```python
from build123d import *

# Parameters (mm, degrees)
SKETCH1_W           = 90
SKETCH1_H           = 45
BOSS_EXTRUDE1_DEPTH = 50
SKETCH2_R           = 4.15
CUT_EXTRUDE1_DEPTH  = 28.296664924
SKETCH3_R           = 4.15
CUT_EXTRUDE2_DEPTH  = 106.386194542


with BuildPart() as part:
    # Sketch1 → Boss-Extrude1 (new body)
    with BuildSketch(Plane(origin=(0, 0, 0), x_dir=(1, 0, 0), z_dir=(0, 1, 0))):
        Rectangle(SKETCH1_W, SKETCH1_H)
    extrude(amount=BOSS_EXTRUDE1_DEPTH)

    # Sketch2 → Cut-Extrude1 (cut)
    with BuildSketch(Plane.XY.offset(22.5)):
        with Locations((-30, 37.5)):
            Circle(SKETCH2_R)
        with Locations(Location((30, 37.5, 0), (0, 0, 180))):
            Circle(SKETCH2_R)
    extrude(amount=-CUT_EXTRUDE1_DEPTH, mode=Mode.SUBTRACT)

    # Sketch3 → Cut-Extrude2 (cut, through all)
    with BuildSketch(Plane(origin=(45, 0, 0), x_dir=(0, 0, -1), z_dir=(1, 0, 0))):
        with Locations((0, 12.5)):
            Circle(SKETCH3_R)
    extrude(amount=-CUT_EXTRUDE2_DEPTH, mode=Mode.SUBTRACT)


solid = part.part
```
Verification items for the finished model (mm, model axes). A direction names the side the tool comes from. Round coordinates to 2 decimals unless told otherwise and drop trailing zeros. Order: outer loops, then holes, each group sorted by start corner. A loop starts at its lowest first (then second) coordinate and runs counter-clockwise, first axis right, second up.
1) Material ranges on line 1 (Y direction, x = -30, z = 8.25); line 2 (X direction, y = 36, z = 11); line 3 (X direction, y = 39.5, z = 11.5), recorded low to high.
Geometry says:
line 1: y = 0 to 33.35, 41.65 to 50
line 2: x = -45 to -33.87, -26.13 to 26.13, 33.87 to 45
line 3: x = -45 to -33.64, -26.36 to 26.36, 33.64 to 45
2) Draft check along X on faces 3 (the flat face through (-1, 25, -22.5)), 4 (the flat face through (-30, 38, -5.797)), 5 (the flat face through (-45, 25, 0)), 6 (the flat face through (45, 25, 0)). Enter one of: +X half, -X half, draft (parallel to the pull), parting line (faces both ways), or undercut.
Geometry says:
face 3: draft
face 4: undercut
face 5: -X half
face 6: +X half
3) Cross-section at B-B, the plane y = 12.5. Record the cut outline in (x, z).
Geometry says:
outline: (-45, -22.5) - (45, -22.5) - (45, -4.15) - (-45, -4.15) - close; (-45, 4.15) - (45, 4.15) - (45, 22.5) - (-45, 22.5) - close
4) Cross-section at D-D, the plane z = 8.5. Record the cut outline in (x, y).
Geometry says:
outline: (-45, 0) - (45, 0) - (45, 50) - (-45, 50) - close; hole circle Ø8.3 at (-30, 37.5); hole circle Ø8.3 at (30, 37.5)
5) Cross-section at A-A, the plane z = 0. Record the cut outline in (x, y), plus the area to 3 significant figures.
Geometry says:
outline: (-45, 0) - (45, 0) - (45, 8.35) - (-45, 8.35) - close; (-45, 16.65) - (45, 16.65) - (45, 50) - (-45, 50) - close; hole circle Ø8.3 at (-30, 37.5); hole circle Ø8.3 at (30, 37.5)
area: 3,640 mm2
6) Cross-section at C-C, the plane x = 30. Record the cut outline in (y, z).
Geometry says:
outline: (0, -22.5) - (50, -22.5) - (50, 22.5) - (41.65, 22.5) - (41.65, -5.8) - (33.35, -5.8) - (33.35, 22.5) - (0, 22.5) - close; hole circle Ø8.3 at (12.5, 0)
7) Depth check by flat-ended pin: pin 1 (7.5 mm diameter, centred on x = -30, y = 37.5, fed in from +Z). Enter the tip coordinate at first touch or a pass-through.
Geometry says:
pin 1: stops at z = -5.8
8) Tool access check on faces 1 (the flat face through (-1, 0, 0)), 2 (the cylindrical face through (-27.77, 41, 8.55)). Record the directions out of +Z, -Z, +X, -X, +Y, -Y that give a thin tool (end or side, any length) a straight path to the whole face; none if there is none.
Geometry says:
face 1: +Z, -Z, +X, -X, -Y
face 2: +Z
